Input: part model. Units: mm. Frame: model coordinates. Face numbers are marked on the shaded views. A direction names the side the tool comes from. Give positions to 0.01 mm unless a question says otherwise; leave off trailing zeros. Order: outer loops, then holes, each group sorted by start corner. A loop starts at its lowest first (then second) coordinate and runs counter-clockwise, first axis right, second up. Notation, with made-up numbers: (39.5, 79) - (91.5, 79) arc R16 ccw to (91.5, 110) - close; hole circle Ø1 at (36.25, 79.25). An arc over 180 degrees is marked (long way). Answer in a Markdown table with one row per item. Add a question column.
1. Section query A-A on x = -1. Return loops of the section in (y, z), and give its area (3 significant figures).
2. Access query for the marked faces 5, 6, 7 and 8. Directions: +Z, -Z, +X, -X, +Y, -Y. A direction counts if a zero-diameter tool reaches every point of the face in a straight line with its end or side. Return the directions, or none.
3. Contact query for flat-ended pins moving along their axis: pin 1 (1 mm diameter, centred on y = 7.5, z = 13.5, fed in from -X); pin 2 (2 mm diameter, centred on y = 5.5, z = -8, fed in from +X); pin 3 (2 mm diameter, centred on y = 1.5, z = 3.5, fed in from -X). Output: stop coordinate, or through.
4. Section query D-D on x = 10.5. Return loops of the section in (y, z), and give its area (3 significant figures).
5. Ray query, line 1 (Z direction, x = -17.5, y = 10.75); line 2 (Z direction, x = 0, y = 8); line 3 (X direction, y = 1.25, z = -16.5). Return the intervals inside material, ascending. Write a range as [from, to].
6. Section query C-C on x = -6. Return loops of the section in (y, z).
7. Mould query, pull axis X, two halves, no side actions, for the marked faces 1, 2, 3 and 4. Classes: released by +X, released by -X, zero draft, split by the parting line, or undercut.
8. Section query B-B on z = -10.5. Return loops of the section in (x, y), and give its area (3 significant figures).
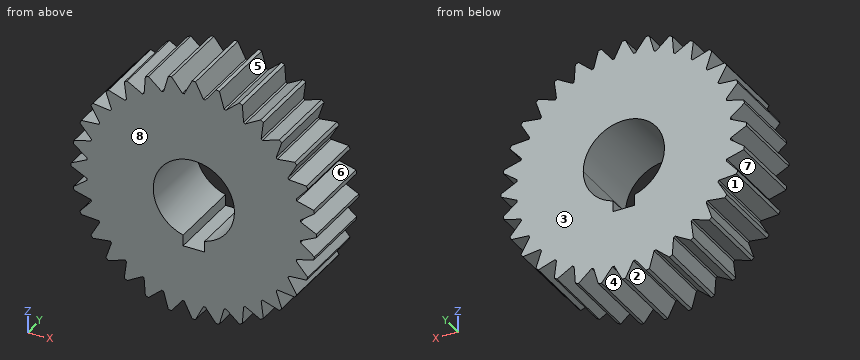
```python
from build123d import *

# Parameters (mm, degrees)
BOSS_EXTRUDE1_DEPTH = 12.7
SKETCH2_OUTSIDE_W   = 55.852
SKETCH2_OUTSIDE_H   = 55.852
SKETCH2_OUTSIDE_R   = 20.32
CUT_EXTRUDE1_DEPTH  = 33.149212754
CUT_EXTRUDE3_DEPTH  = 32.418064867


with BuildPart() as part:
    # Sketch1 → Boss-Extrude1 (new body)
    with BuildSketch(Plane(origin=(0, 0, 0), x_dir=(1, 0, 0), z_dir=(0, 1, 0))):
        with BuildLine():
            Line((0, 20.883987655), (-1.5875, 17.708987655))
            ThreePointArc((-1.5875, 17.708987655), (-1.742744755, 17.69438444), (-1.897855471, 17.678420309))
            Line((-1.897855471, 17.678420309), (-4.074263877, 20.482707688))
            Line((-4.074263877, 20.482707688), (-5.011848737, 17.059008536))
            ThreePointArc((-5.011848737, 17.059008536), (-5.161261562, 17.014399169), (-5.310277422, 16.968481184))
            Line((-5.310277422, 16.968481184), (-7.991956077, 19.294288751))
            Line((-7.991956077, 19.294288751), (-8.243594937, 15.753461287))
            ThreePointArc((-8.243594937, 15.753461287), (-8.381433981, 15.68056008), (-8.518628388, 15.606452844))
            Line((-8.518628388, 15.606452844), (-11.602521888, 17.364401118))
            Line((-11.602521888, 17.364401118), (-11.158544407, 13.842517355))
            ThreePointArc((-11.158544407, 13.842517355), (-11.279512592, 13.744125861), (-11.399613243, 13.644677274))
            Line((-11.399613243, 13.644677274), (-14.767209289, 14.767209289))
            Line((-14.767209289, 14.767209289), (-13.644677274, 11.399613243))
            ThreePointArc((-13.644677274, 11.399613243), (-13.744125861, 11.279512592), (-13.842517355, 11.158544407))
            Line((-13.842517355, 11.158544407), (-17.364401118, 11.602521888))
            Line((-17.364401118, 11.602521888), (-15.606452844, 8.518628388))
            ThreePointArc((-15.606452844, 8.518628388), (-15.68056008, 8.381433981), (-15.753461287, 8.243594937))
            Line((-15.753461287, 8.243594937), (-19.294288751, 7.991956077))
            Line((-19.294288751, 7.991956077), (-16.968481184, 5.310277422))
            ThreePointArc((-16.968481184, 5.310277422), (-17.014399169, 5.161261562), (-17.059008536, 5.011848737))
            Line((-17.059008536, 5.011848737), (-20.482707688, 4.074263877))
            Line((-20.482707688, 4.074263877), (-17.678420309, 1.897855471))
            ThreePointArc((-17.678420309, 1.897855471), (-17.69438444, 1.742744755), (-17.708987655, 1.5875))
            Line((-17.708987655, 1.5875), (-20.883987655, 0))
            Line((-20.883987655, 0), (-17.708987655, -1.5875))
            ThreePointArc((-17.708987655, -1.5875), (-17.69438444, -1.742744755), (-17.678420309, -1.897855471))
            Line((-17.678420309, -1.897855471), (-20.482707688, -4.074263877))
            Line((-20.482707688, -4.074263877), (-17.059008536, -5.011848737))
            ThreePointArc((-17.059008536, -5.011848737), (-17.014399169, -5.161261562), (-16.968481184, -5.310277422))
            Line((-16.968481184, -5.310277422), (-19.294288751, -7.991956077))
            Line((-19.294288751, -7.991956077), (-15.753461287, -8.243594937))
            ThreePointArc((-15.753461287, -8.243594937), (-15.68056008, -8.381433981), (-15.606452844, -8.518628388))
            Line((-15.606452844, -8.518628388), (-17.364401118, -11.602521888))
            Line((-17.364401118, -11.602521888), (-13.842517355, -11.158544407))
            ThreePointArc((-13.842517355, -11.158544407), (-13.744125861, -11.279512592), (-13.644677274, -11.399613243))
            Line((-13.644677274, -11.399613243), (-14.767209289, -14.767209289))
            Line((-14.767209289, -14.767209289), (-11.399613243, -13.644677274))
            ThreePointArc((-11.399613243, -13.644677274), (-11.279512592, -13.744125861), (-11.158544407, -13.842517355))
            Line((-11.158544407, -13.842517355), (-11.602521888, -17.364401118))
            Line((-11.602521888, -17.364401118), (-8.518628388, -15.606452844))
            ThreePointArc((-8.518628388, -15.606452844), (-8.381433981, -15.68056008), (-8.243594937, -15.753461287))
            Line((-8.243594937, -15.753461287), (-7.991956077, -19.294288751))
            Line((-7.991956077, -19.294288751), (-5.310277422, -16.968481184))
            ThreePointArc((-5.310277422, -16.968481184), (-5.161261562, -17.014399169), (-5.011848737, -17.059008536))
            Line((-5.011848737, -17.059008536), (-4.074263877, -20.482707688))
            Line((-4.074263877, -20.482707688), (-1.897855471, -17.678420309))
            ThreePointArc((-1.897855471, -17.678420309), (-1.742744755, -17.69438444), (-1.5875, -17.708987655))
            Line((-1.5875, -17.708987655), (0, -20.883987655))
            Line((0, -20.883987655), (1.5875, -17.708987655))
            ThreePointArc((1.5875, -17.708987655), (1.742744755, -17.69438444), (1.897855471, -17.678420309))
            Line((1.897855471, -17.678420309), (4.074263877, -20.482707688))
            Line((4.074263877, -20.482707688), (5.011848737, -17.059008536))
            ThreePointArc((5.011848737, -17.059008536), (5.161261562, -17.014399169), (5.310277422, -16.968481184))
            Line((5.310277422, -16.968481184), (7.991956077, -19.294288751))
            Line((7.991956077, -19.294288751), (8.243594937, -15.753461287))
            ThreePointArc((8.243594937, -15.753461287), (8.381433981, -15.68056008), (8.518628388, -15.606452844))
            Line((8.518628388, -15.606452844), (11.602521888, -17.364401118))
            Line((11.602521888, -17.364401118), (11.158544407, -13.842517355))
            ThreePointArc((11.158544407, -13.842517355), (11.279512592, -13.744125861), (11.399613243, -13.644677274))
            Line((11.399613243, -13.644677274), (14.767209289, -14.767209289))
            Line((14.767209289, -14.767209289), (13.644677274, -11.399613243))
            ThreePointArc((13.644677274, -11.399613243), (13.744125861, -11.279512592), (13.842517355, -11.158544407))
            Line((13.842517355, -11.158544407), (17.364401118, -11.602521888))
            Line((17.364401118, -11.602521888), (15.606452844, -8.518628388))
            ThreePointArc((15.606452844, -8.518628388), (15.68056008, -8.381433981), (15.753461287, -8.243594937))
            Line((15.753461287, -8.243594937), (19.294288751, -7.991956077))
            Line((19.294288751, -7.991956077), (16.968481184, -5.310277422))
            ThreePointArc((16.968481184, -5.310277422), (17.014399169, -5.161261562), (17.059008536, -5.011848737))
            Line((17.059008536, -5.011848737), (20.482707688, -4.074263877))
            Line((20.482707688, -4.074263877), (17.678420309, -1.897855471))
            ThreePointArc((17.678420309, -1.897855471), (17.69438444, -1.742744755), (17.708987655, -1.5875))
            Line((17.708987655, -1.5875), (20.883987655, 0))
            Line((20.883987655, 0), (17.708987655, 1.5875))
            ThreePointArc((17.708987655, 1.5875), (17.69438444, 1.742744755), (17.678420309, 1.897855471))
            Line((17.678420309, 1.897855471), (20.482707688, 4.074263877))
            Line((20.482707688, 4.074263877), (17.059008536, 5.011848737))
            ThreePointArc((17.059008536, 5.011848737), (17.014399169, 5.161261562), (16.968481184, 5.310277422))
            Line((16.968481184, 5.310277422), (19.294288751, 7.991956077))
            Line((19.294288751, 7.991956077), (15.753461287, 8.243594937))
            ThreePointArc((15.753461287, 8.243594937), (15.68056008, 8.381433981), (15.606452844, 8.518628388))
            Line((15.606452844, 8.518628388), (17.364401118, 11.602521888))
            Line((17.364401118, 11.602521888), (13.842517355, 11.158544407))
            ThreePointArc((13.842517355, 11.158544407), (13.744125861, 11.279512592), (13.644677274, 11.399613243))
            Line((13.644677274, 11.399613243), (14.767209289, 14.767209289))
            Line((14.767209289, 14.767209289), (11.399613243, 13.644677274))
            ThreePointArc((11.399613243, 13.644677274), (11.279512592, 13.744125861), (11.158544407, 13.842517355))
            Line((11.158544407, 13.842517355), (11.602521888, 17.364401118))
            Line((11.602521888, 17.364401118), (8.518628388, 15.606452844))
            ThreePointArc((8.518628388, 15.606452844), (8.381433981, 15.68056008), (8.243594937, 15.753461287))
            Line((8.243594937, 15.753461287), (7.991956077, 19.294288751))
            Line((7.991956077, 19.294288751), (5.310277422, 16.968481184))
            ThreePointArc((5.310277422, 16.968481184), (5.161261562, 17.014399169), (5.011848737, 17.059008536))
            Line((5.011848737, 17.059008536), (4.074263877, 20.482707688))
            Line((4.074263877, 20.482707688), (1.897855471, 17.678420309))
            ThreePointArc((1.897855471, 17.678420309), (1.742744755, 17.69438444), (1.5875, 17.708987655))
            Line((1.5875, 17.708987655), (0, 20.883987655))
        make_face()
    extrude(amount=BOSS_EXTRUDE1_DEPTH)

    # Sketch2 outside → Cut-Extrude1 (cut, through all)
    with BuildSketch(Plane(origin=(0, 12.7, 0), x_dir=(1, 0, 0), z_dir=(0, 1, 0))):
        Rectangle(SKETCH2_OUTSIDE_W, SKETCH2_OUTSIDE_H)
        Circle(SKETCH2_OUTSIDE_R, mode=Mode.SUBTRACT)
    extrude(amount=-CUT_EXTRUDE1_DEPTH, mode=Mode.SUBTRACT)

    # Sketch3 → Cut-Extrude3 (cut, through all)
    with BuildSketch(Plane(origin=(0, 12.7, 0), x_dir=(1, 0, 0), z_dir=(0, 1, 0))):
        with BuildLine():
            ThreePointArc((1.778, 6.491923983), (0, 6.731), (-1.778, 6.491923983))
            Line((-1.778, 6.491923983), (-1.778, 5.1435))
            Line((-1.778, 5.1435), (1.778, 5.1435))
            Line((1.778, 5.1435), (1.778, 6.491923983))
        make_face()
        with BuildLine():
            Line((-1.778, 5.1435), (-1.778, 6.491923983))
            ThreePointArc((-1.778, 6.491923983), (-4.082808041, -5.351358659), (6.731, 0))
            ThreePointArc((6.731, 0), (5.351358659, 4.082808041), (1.778, 6.491923983))
            Line((1.778, 6.491923983), (1.778, 5.1435))
            Line((1.778, 5.1435), (-1.778, 5.1435))
        make_face()
        with BuildLine():
            Line((1.778, 8.3185), (-1.778, 8.3185))
            Line((-1.778, 8.3185), (-1.778, 6.491923983))
            ThreePointArc((-1.778, 6.491923983), (0, 6.731), (1.778, 6.491923983))
            Line((1.778, 6.491923983), (1.778, 8.3185))
        make_face()
    extrude(amount=-CUT_EXTRUDE3_DEPTH, mode=Mode.SUBTRACT)


solid = part.part
```
Answer:
| question | item | result |
|---|---|---|
| 1 | outline | (0, -18.88) - (12.7, -18.88) - (12.7, -8.32) - (0, -8.32) - close; (0, 6.66) - (12.7, 6.66) - (12.7, 18.88) - (0, 18.88) - close |
| 1 | area | 289 mm² |
| 2 | face 5 | +Z, +Y, -Y |
| 2 | face 6 | +X, +Y, -Y |
| 2 | face 7 | -X, +Y, -Y |
| 2 | face 8 | +Z, -Z, +X, -X, -Y |
| 3 | pin 1 | stops at x = -14.51 |
| 3 | pin 2 | stops at x = 18.88 |
| 3 | pin 3 | stops at x = -19.98 |
| 4 | outline | (0, -16.74) - (12.7, -16.74) - (12.7, 16.74) - (0, 16.74) - close |
| 4 | area | 425 mm² |
| 5 | line 1 | z = [-8.12, -5.92], [-4.89, 4.89], [5.92, 8.12] |
| 5 | line 2 | z = [-20.32, -8.32], [6.73, 20.32] |
| 5 | line 3 | x = [-11.49, -10.09], [-8.19, 8.19], [10.09, 11.49] |
| 6 | outline | (0, -17.57) - (12.7, -17.57) - (12.7, -3.05) - (0, -3.05) - close; (0, 3.05) - (12.7, 3.05) - (12.7, 17.57) - (0, 17.57) - close |
| 7 | face 1 | released by -X |
| 7 | face 2 | undercut |
| 7 | face 3 | zero draft |
| 7 | face 4 | undercut |
| 8 | outline | (-16.74, 0) - (16.74, 0) - (16.74, 12.7) - (-16.74, 12.7) - close |
| 8 | area | 425 mm² |
